```python
from build123d import *

# Parameters (mm, degrees)
SKETCH2_W                   = 500
SKETCH2_H                   = 185
BASE_DEPTH                  = 4
SKETCH3_W                   = 20
SKETCH3_H                   = 4
TOP_HOLE_DEFINITION_DEPTH   = 267.593792126
TOP_HOLE_PATTERN_COUNT      = 5
TOP_HOLE_PATTERN_PITCH      = 55
TOP_HOLE_PATTERN_COL_COUNT  = 5
TOP_HOLE_PATTERN_COL_PITCH  = 55
SKETCH4_W                   = 4
SKETCH4_H                   = 20
LEFT_HOLE_DEFINITION_DEPTH  = 267.593792126
LEFT_HOLE_PATTERN_COUNT     = 2
LEFT_HOLE_PATTERN_PITCH     = 55
LEFT_HOLE_PATTERN_COL_COUNT = 2
LEFT_HOLE_PATTERN_COL_PITCH = 55
FILLET1_R                   = 10
MIRROR2_COPY_1_SKETCH_W     = 4
MIRROR2_COPY_1_SKETCH_H     = 20
MIRROR2_COPY_1_DEPTH        = 267.593792126
MIRROR2_COPY_2_SKETCH_W     = 4
MIRROR2_COPY_2_SKETCH_H     = 20
MIRROR2_COPY_2_DEPTH        = 267.593792126
SKETCH7_R                   = 8
SKETCH7_R_2                 = 10
CUT_EXTRUDE5_DEPTH          = 267.593792126


with BuildPart() as part:
    # Sketch2 → Base (new body)
    with BuildSketch(Plane(origin=(0, 0, 0), x_dir=(1, 0, 0), z_dir=(0, 1, 0))):
        Rectangle(SKETCH2_W, SKETCH2_H)
    extrude(amount=BASE_DEPTH)

    # Sketch3 → Top Hole Definition (cut, through all)
    with BuildSketch(Plane(origin=(0, 4, 0), x_dir=(1, 0, 0), z_dir=(0, 1, 0))):
        with Locations((0, 85.5)):
            Rectangle(SKETCH3_W, SKETCH3_H)
    top_hole_definition = extrude(amount=-TOP_HOLE_DEFINITION_DEPTH, mode=Mode.SUBTRACT)

    # Top Hole Pattern: Top Hole Definition ×5
    with Locations(*[(-i * TOP_HOLE_PATTERN_PITCH, 0, 0) for i in range(1, TOP_HOLE_PATTERN_COUNT)]):
        add(top_hole_definition, mode=Mode.SUBTRACT)

    # Top Hole Pattern col: Top Hole Definition ×5
    with Locations(*[(i * TOP_HOLE_PATTERN_COL_PITCH, 0, 0) for i in range(1, TOP_HOLE_PATTERN_COL_COUNT)]):
        add(top_hole_definition, mode=Mode.SUBTRACT)

    # Sketch4 → Left Hole Definition (cut, through all)
    with BuildSketch(Plane(origin=(0, 4, 0), x_dir=(1, 0, 0), z_dir=(0, 1, 0))):
        with Locations((-243, 0)):
            Rectangle(SKETCH4_W, SKETCH4_H)
    left_hole_definition = extrude(amount=-LEFT_HOLE_DEFINITION_DEPTH, mode=Mode.SUBTRACT)

    # Left Hole Pattern: Left Hole Definition ×2
    with Locations(*[(0, 0, -i * LEFT_HOLE_PATTERN_PITCH) for i in range(1, LEFT_HOLE_PATTERN_COUNT)]):
        add(left_hole_definition, mode=Mode.SUBTRACT)

    # Left Hole Pattern col: Left Hole Definition ×2
    with Locations(*[(0, 0, i * LEFT_HOLE_PATTERN_COL_PITCH) for i in range(1, LEFT_HOLE_PATTERN_COL_COUNT)]):
        add(left_hole_definition, mode=Mode.SUBTRACT)

    # Fillet1
    fillet1_edges = [part.edges().sort_by_distance(p)[0] for p in [
        (-250, 2, -92.5),
        (250, 2, -92.5),
        (250, 2, 92.5),
        (-250, 2, 92.5),
    ]]
    fillet(fillet1_edges, radius=FILLET1_R)

    # Mirror2: Left Hole Definition across plane
    add(left_hole_definition.mirror(Plane(origin=(0, 0, 0), x_dir=(0, 0, 1), z_dir=(1, 0, 0))), mode=Mode.SUBTRACT)

    # Mirror2 copy 1 sketch → Mirror2 copy 1 (cut, through all)
    with BuildSketch(Plane(origin=(0, 4, -55), x_dir=(-1, 0, 0), z_dir=(0, 1, 0))):
        with Locations((-243, 0)):
            Rectangle(MIRROR2_COPY_1_SKETCH_W, MIRROR2_COPY_1_SKETCH_H)
    extrude(amount=-MIRROR2_COPY_1_DEPTH, mode=Mode.SUBTRACT)

    # Mirror2 copy 2 sketch → Mirror2 copy 2 (cut, through all)
    with BuildSketch(Plane(origin=(0, 4, 55), x_dir=(-1, 0, 0), z_dir=(0, 1, 0))):
        with Locations((-243, 0)):
            Rectangle(MIRROR2_COPY_2_SKETCH_W, MIRROR2_COPY_2_SKETCH_H)
    extrude(amount=-MIRROR2_COPY_2_DEPTH, mode=Mode.SUBTRACT)

    # Sketch7 → Cut-Extrude5 (cut, through all)
    with BuildSketch(Plane.XZ):
        with Locations(Location((-209, 59.798294078, 0), (0, 0, 270))):
            Circle(SKETCH7_R)
        with Locations(Location((-168, 59.798294078, 0), (0, 0, 270))):
            Circle(SKETCH7_R)
        with Locations(Location((-127, 59.798294078, 0), (0, 0, 270))):
            Circle(SKETCH7_R)
        with Locations(Location((-86, 59.798294078, 0), (0, 0, 270))):
            Circle(SKETCH7_R)
        with Locations(Location((-45, 59.798294078, 0), (0, 0, 270))):
            Circle(SKETCH7_R)
        with Locations(Location((-4, 59.798294078, 0), (0, 0, 270))):
            Circle(SKETCH7_R)
        with Locations(Location((37, 59.798294078, 0), (0, 0, 270))):
            Circle(SKETCH7_R)
        with Locations(Location((78, 59.798294078, 0), (0, 0, 270))):
            Circle(SKETCH7_R)
        with Locations(Location((-179.5, 9.310158007, 0), (0, 0, 270))):
            Circle(SKETCH7_R_2)
        with Locations(Location((-209, 6.747125767, 0), (0, 0, 270))):
            Circle(SKETCH7_R)
        with Locations(Location((157.298294078, 61.5, 0), (0, 0, 270))):
            Circle(SKETCH7_R)
        with Locations(Location((157.431778922, 37.500371215, 0), (0, 0, 270))):
            Circle(SKETCH7_R)
        with Locations(Location((157.565263767, 13.500742431, 0), (0, 0, 270))):
            Circle(SKETCH7_R)
        with Locations(Location((157.698748611, -10.498886354, 0), (0, 0, 270))):
            Circle(SKETCH7_R)
    extrude(amount=-CUT_EXTRUDE5_DEPTH, mode=Mode.SUBTRACT)


solid = part.part
```
Geometry: final body of the model. Coordinates: model frame, mm. Round coordinates to 2 decimals unless told otherwise and drop trailing zeros. Order: outer loops, then holes, each group sorted by start corner. A loop starts at its lowest first (then second) coordinate and runs counter-clockwise, first axis right, second up. Notation, with made-up numbers: (-8.5, 5) -> (42.5, 5) arc R20 ccw to (42.5, 40) -> close; hole circle Ø2 at (45, -12.5). An arc over 180 degrees is marked (long way). Write each question's results on one line, items separated by ' | '.
Q1. Ray query, line 1 along X through (y, z) = (3.25, 50); line 2 along Z through (x, y) = (150.5, 2.6); line 3 along X through (y, z) = (0.7, 9.5). Return the intervals inside material, ascending.
Response values:
line 1: -250 to -245, -241 to 241, 245 to 250 | line 2: -92.5 to -13.99, -7.01 to 9.75, 17.25 to 33.51, 41.49 to 57.28, 65.72 to 92.5 | line 3: -250 to -245, -241 to -216.51, -201.49 to -189.5, -169.5 to 150.64, 164.49 to 241, 245 to 250
Q2. Pull-direction query (X, two-part tool) for faces 1 (the face through (-247.15, 2.03, 89.49)), 2 (the face through (-3, 0, -1)), 3 (the face through (-1.597, 1.972, 52.168)); classes: released by +X, released by -X, zero draft, split by the parting line, or undercut.
Response values:
face 1: released by -X | face 2: zero draft | face 3: undercut
Q3. Pin query (flat end, axial travel): pin 1 Ø1.2 at (x, y) = (-242.5, 1) entering from -Z; pin 2 Ø2 at (x, y) = (242.5, 1.5) entering from +Z. Return the tip coordinate at first contact, or that it passes through.
Response values:
pin 1: z = -92.32 | pin 2: z = 92.39
Q4. Section query B-B (x = -4). Output: boundary loops of the cut face in (y, z).
Response values:
outline: (0, -92.5) -> (4, -92.5) -> (4, -87.5) -> (0, -87.5) -> close; (0, -83.5) -> (4, -83.5) -> (4, 51.8) -> (0, 51.8) -> close; (0, 67.8) -> (4, 67.8) -> (4, 92.5) -> (0, 92.5) -> close
Q5. Section query A-A (x = 78). Output: boundary loops of the cut face in (y, z), and give its area (3 significant figures).
Response values:
outline: (0, -92.5) -> (4, -92.5) -> (4, 51.8) -> (0, 51.8) -> close; (0, 67.8) -> (4, 67.8) -> (4, 92.5) -> (0, 92.5) -> close | area: 676 mm²
Q6. Section query C-C (y = 0.75). Count the separate pieces of the cut face and the enclosed holes in it, and give its area (3 significant figures).
Response values:
separate pieces: 1 | enclosed holes: 29 | area: 88,300 mm²
